Part model, mm, in its own coordinate system. Give positions to 0.01 mm unless a question says otherwise; leave off trailing zeros. Order: outer loops, then holes, each group sorted by start corner. A loop starts at its lowest first (then second) coordinate and runs counter-clockwise, first axis right, second up. Notation, with made-up numbers: M 61,-33 L 111,-33 A18 ccw 111,-12 Z; hole C 10,-39 d9. An arc over 180 degrees is marked long. Answer as a JSON object with one key per item and string values.
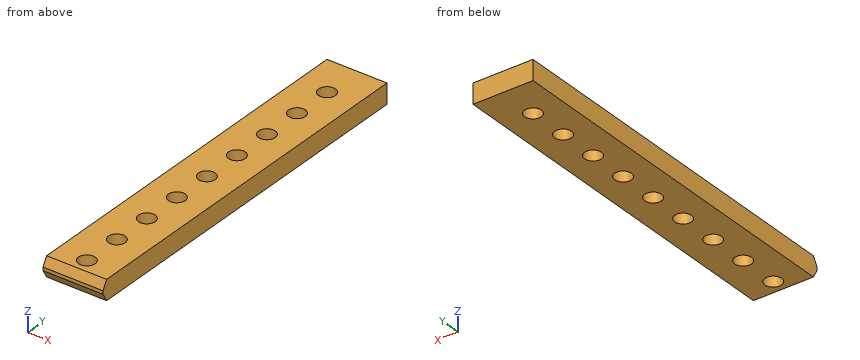
from build123d import *

# Parameters (mm, degrees)
SKETCH_1_W          = 75
SKETCH_1_H          = 473
EXTRUDE_1_DEPTH     = 25
SKETCH_2_R          = 10.5
CUT_EXTRUDE_1_DEPTH = 26
CHAMFER_1_SIZE      = 6
CHAMFER_1_SIZE2     = 10.392304845
CHAMFER_2_SIZE      = 6
CHAMFER_2_SIZE2     = 10.392304845


with BuildPart() as part:
    # Эскиз1 → Бобышка-Вытянуть1 (new body)
    with BuildSketch(Plane.XY):
        with Locations((37.5, 236.5)):
            Rectangle(SKETCH_1_W, SKETCH_1_H)
    extrude(amount=EXTRUDE_1_DEPTH)

    # Эскиз2 → Вырез-Вытянуть1 (cut, through all)
    with BuildSketch(Plane.XY.offset(25)):
        with Locations((37.5, 23)):
            Circle(SKETCH_2_R)
        with Locations((37.5, 73)):
            Circle(SKETCH_2_R)
        with Locations((37.5, 123)):
            Circle(SKETCH_2_R)
        with Locations((37.5, 173)):
            Circle(SKETCH_2_R)
        with Locations((37.5, 223)):
            Circle(SKETCH_2_R)
        with Locations((37.5, 273)):
            Circle(SKETCH_2_R)
        with Locations((37.5, 323)):
            Circle(SKETCH_2_R)
        with Locations((37.5, 373)):
            Circle(SKETCH_2_R)
        with Locations((37.5, 423)):
            Circle(SKETCH_2_R)
    extrude(amount=-CUT_EXTRUDE_1_DEPTH, mode=Mode.SUBTRACT)

    # Фаска1
    chamfer_1_edges = [part.edges().sort_by_distance(p)[0] for p in [
        (37.5, 0, 0),
    ]]
    chamfer_1_side = [part.faces().sort_by_distance(p)[0] for p in [
        (37.5, 237.800547955, 0),
    ]]
    chamfer(chamfer_1_edges, length=CHAMFER_1_SIZE, length2=CHAMFER_1_SIZE2, reference=chamfer_1_side[0])

    # Фаска2
    chamfer_2_edges = [part.edges().sort_by_distance(p)[0] for p in [
        (37.5, 0, 25),
    ]]
    chamfer_2_side = [part.faces().sort_by_distance(p)[0] for p in [
        (37.5, 237.800547955, 25),
    ]]
    chamfer(chamfer_2_edges, length=CHAMFER_2_SIZE, length2=CHAMFER_2_SIZE2, reference=chamfer_2_side[0])


solid = part.part
1. Probe line 1 along X through (y, z) = (222.5, 2); line 2 along X through (y, z) = (68, 4.5); line 3 along Y through (x, z) = (58.5, 8.75). List the from-to ranges inside material, lowest first.
Worked answers:
{"line 1": "x = 0 to 27.01, 47.99 to 75", "line 2": "x = 0 to 28.27, 46.73 to 75", "line 3": "y = 0.95 to 473"}
2. Cut at B-B on x = 37.5. State how many separate pieces and enclosed holes the cut face has, plus the area to 3 significant figures.
Worked answers:
{"separate pieces": "10", "enclosed holes": "0", "area": "7,040 mm^2"}
3. Pin check, flat tips, straight feed: P1, Ø12, axis at x = 40, y = 371, coming from the -Z side (3 decimals); P2, Ø8, axis at x = 10, z = 20.5, coming from the -Y side; P3, Ø8, axis at x = 36, y = 265.5, coming from the -Z side; P4, Ø2, axis at x = 60.5, z = 21.5, coming from the -Y side. Stop position of each tip, or through.
Worked answers:
{"P1": "passes through", "P2": "stops at y = 1.09", "P3": "stops at z = 0", "P4": "stops at y = 3.4"}
4. Cut at A-A on y = 73. Give the cut face in (x, z).
Worked answers:
{"outline": "M 0,0 L 27,0 L 27,25 L 0,25 Z; M 48,0 L 75,0 L 75,25 L 48,25 Z"}
